Check sheet for the modelled part. Datum: model origin and axes. Units: mm. A direction names the side the tool comes from. Give positions to 0.01 mm unless a question says otherwise; leave off trailing zeros. Order: outer loops, then holes, each group sorted by start corner. A loop starts at its lowest first (then second) coordinate and runs counter-clockwise, first axis right, second up.
```python
from build123d import *

# Parameters (mm, degrees)
F0_R          = 24
F0_R_2        = 8
F1_DEPTH      = 5
F2_DEPTH      = 11
F3_R          = 2.5
F4_DEPTH      = 0.5
F5_R          = 1.5
F6_DEPTH      = 25
F5_R_2        = 1
F7_DEPTH      = 8
F8_R          = 1.5
F9_DEPTH      = 24.001
F9_DEPTH_BACK = 24.001


with BuildPart() as f1:
    # F0 (on Front) → F1 (new body)
    with BuildSketch(Plane.XZ):
        Circle(F0_R)
        Circle(F0_R_2, mode=Mode.SUBTRACT)
        Circle(F0_R_2)
    extrude(amount=F1_DEPTH)

    # F0 (on Front) → F2 (join)
    with BuildSketch(Plane.XZ):
        Circle(F0_R_2)
    extrude(amount=-F2_DEPTH)

    # F3 (on face) → F4 (join)
    with BuildSketch(Plane(origin=(0, 11, 0), x_dir=(-1, 0, 0), z_dir=(0, 1, 0))):
        Circle(F3_R)
    extrude(amount=F4_DEPTH)

    # F5 (on face) → F6 (cut)
    with BuildSketch(Plane.XZ.offset(5)):
        Circle(F5_R)
    extrude(amount=-F6_DEPTH, mode=Mode.SUBTRACT)

    # F5 (on face) → F7 (join)
    with BuildSketch(Plane.XZ.offset(5)):
        with Locations((0, 4)):
            Circle(F5_R_2)
    extrude(amount=F7_DEPTH)

    # F8 (on Right) → F9 (cut, two sides)
    with BuildSketch(Plane.YZ) as f9_sk:
        with Locations((7, 0)):
            Circle(F8_R)
    extrude(amount=-F9_DEPTH, mode=Mode.SUBTRACT)
    extrude(f9_sk.sketch, amount=F9_DEPTH_BACK, mode=Mode.SUBTRACT)


solid = f1.part
```
(1) Sectioned sample at D-D (y = -3). Enter the section's corners in (x, z).
(2) Go/stop test with flat-tipped pins: P1, Ø6, axis at y = -7, z = -5, coming from the -X side; P2, Ø1, axis at x = 19, z = -4, coming from the -Y side; P3, Ø2, axis at x = -14.5, y = -3.5, coming from the -Z side. Record where each tip stops, or that it passes through.
(3) Sectioned sample at A-A (z = 0). Enter the section's corners in (x, y), plus the area to 3 significant figures.
(4) Tool access check on faces 1 (the face through (0, -9, 5)), 2 (the face through (-23.977, -2.465, 1.055)), 3 (the face through (2, 11, 2)). Record the directions out of +Z, -Z, +X, -X, +Y, -Y that give a thin tool (end or side, any length) a straight path to the whole face; none if there is none.
(5) Release check for a two-part mould opening along Z. For faces 4 (the face through (0.54, 11.25, -2.44)), 5 (the face through (4.83, 5.5, 0.07)), 6 (the face through (5, -5, 0)) record: released by +Z, released by -Z, zero draft, split by the parting line, or undercut.
(6) Sectioned sample at C-C (x = -6). Enter the section's corners in (y, z).
(7) Thickness scan on L1, parallel to Z at x = 0, y = -2; L2, parallel to Z at x = 0, y = 2; L3, parallel to Y at x = 2, z = 0. Record the ranges inside material, lowest first.
(8) Sectioned sample at B-B (y = 10). Enter the section's corners in (x, z), plus the area to 3 significant figures.
Values follow:
1. outline: circle Ø48 at (0, 0); hole circle Ø3 at (0, 0)
2. P1: stops at x = -23.84
2. P2: stops at y = -5
2. P3: stops at z = -19.84
3. outline: (-24, -5) - (-1.5, -5) - (-1.5, 5.5) - (-8, 5.5) - (-8, 0) - (-24, 0) - close; (-8, 8.5) - (-1.5, 8.5) - (-1.5, 11.5) - (-2.5, 11.5) - (-2.5, 11) - (-8, 11) - close; (1.5, -5) - (24, -5) - (24, 0) - (8, 0) - (8, 5.5) - (1.5, 5.5) - close; (1.5, 8.5) - (8, 8.5) - (8, 11) - (2.5, 11) - (2.5, 11.5) - (1.5, 11.5) - close
3. area: 330 mm2
4. face 1: -Y
4. face 2: +Y, -Y
4. face 3: +Y
5. face 4: split by the parting line
5. face 5: undercut
5. face 6: zero draft
6. outline: (-5, -23.24) - (0, -23.24) - (0, -5.29) - (11, -5.29) - (11, 5.29) - (0, 5.29) - (0, 23.24) - (-5, 23.24) - close; hole circle Ø3 at (7, 0)
7. L1: z = -24 to -1.5, 1.5 to 24
7. L2: z = -8 to -1.5, 1.5 to 8
7. L3: y = -5 to 5.5, 8.5 to 11.5
8. outline: circle Ø16 at (0, 0); hole circle Ø3 at (0, 0)
8. area: 194 mm2
